from build123d import *

# Parameters (mm, degrees)
SKETCH_1_W         = 10
SKETCH_1_H         = 10
EXTRUDE_1_DEPTH    = 1
EXTRUDE_2_DEPTH    = 1
SKETCH_4_W         = 12
SKETCH_4_H         = 17
EXTRUDE_4_DEPTH    = 1
SKETCH_5_W         = 12
SKETCH_5_H         = 17
EXTRUDE_5_DEPTH    = 1
HOLE_WIZARD_M2_1_D = 1.6


with BuildPart() as part:
    # 草图1 → 凸台-拉伸1 (new body)
    with BuildSketch(Plane(origin=(0, 0, 0), x_dir=(1, 0, 0), z_dir=(0, 1, 0))):
        with Locations((5, 5)):
            Rectangle(SKETCH_1_W, SKETCH_1_H)
    extrude(amount=EXTRUDE_1_DEPTH)

    # 草图2 → 凸台-拉伸2 (add)
    with BuildSketch(Plane.ZY):
        with BuildLine():
            Line((-9.5, 6.5), (-10, 6.5))
            Line((-10, 6.5), (-10, 0))
            Line((-10, 0), (0, 0))
            Line((0, 0), (0, 6.5))
            Line((0, 6.5), (-0.5, 6.5))
            ThreePointArc((-0.5, 6.5), (-5, 2), (-9.5, 6.5))
        make_face()
    extrude(amount=EXTRUDE_2_DEPTH)

    # 草图4 → 凸台-拉伸4 (add)
    with BuildSketch(Plane.XY):
        with Locations((5, 8.5)):
            Rectangle(SKETCH_4_W, SKETCH_4_H)
    extrude(amount=EXTRUDE_4_DEPTH)

    # 草图5 → 凸台-拉伸5 (add)
    with BuildSketch(Plane(origin=(0, 0, -10), x_dir=(-1, 0, 0), z_dir=(0, 0, -1))):
        with Locations((-5, 8.5)):
            Rectangle(SKETCH_5_W, SKETCH_5_H)
    extrude(amount=EXTRUDE_5_DEPTH)

    # M2 螺纹孔1 (through all)
    with Locations(Plane(origin=(0, 0, -11), x_dir=(-1, 0, 0), z_dir=(0, 0, -1))):
        with Locations((-9, 15.5), (-1, 15.5)):
            Hole(HOLE_WIZARD_M2_1_D / 2)


solid = part.part
Geometry: final body of the model. Coordinates: model frame, mm. A direction names the side the tool comes from. Give positions to 0.01 mm unless a question says otherwise; leave off trailing zeros. Order: outer loops, then holes, each group sorted by start corner. A loop starts at its lowest first (then second) coordinate and runs counter-clockwise, first axis right, second up. Notation, with made-up numbers: (-30, 26.5) - (18, 26.5) arc R27 cw to (18, 62.5) - close; hole circle Ø6 at (40.25, 48.5). An arc over 180 degrees is marked (long way). Use CSV: the item, a comma, the result in double quotes.
1. Section query A-A (x = 1). Output: boundary loops of the cut face in (y, z), plus the area to 3 significant figures.
Answers below:
outline,"(0, -11) - (14.7, -11) - (14.7, -10) - (1, -10) - (1, 0) - (14.7, 0) - (14.7, 1) - (0, 1) - close; (16.3, -11) - (17, -11) - (17, -10) - (16.3, -10) - close; (16.3, 0) - (17, 0) - (17, 1) - (16.3, 1) - close"
area,"40.8 mm2"
2. Contact query for a flat-ended pin moving along its axis: pin 1 (0.5 mm diameter, centred on y = 0.5, z = -3, fed in from +X). Output: stop coordinate, or through.
Answers below:
pin 1,"x = 10"
3. Section query D-D (z = -0.25). Output: boundary loops of the cut face in (x, y).
Answers below:
outline,"(-1, 0) - (10, 0) - (10, 1) - (0, 1) - (0, 6.5) - (-1, 6.5) - close"
4. Access query for faces 1 (the face through (0, 2, -6.2)), 2 (the face through (5.1, 17, -10.5)), 3 (the face through (10, 0.5, -4.9)). Directions: +Z, -Z, +X, -X, +Y, -Y. A direction counts if a zero-diameter tool reaches every point of the face in a straight line with its end or side. Return the directions, or none.
Answers below:
face 1,"+X, +Y"
face 2,"+Z, -Z, +X, -X, +Y"
face 3,"+X, +Y, -Y"
5. Section query C-C (x = 10.25). Output: boundary loops of the cut face in (y, z).
Answers below:
outline,"(0, -11) - (17, -11) - (17, -10) - (0, -10) - close; (0, 0) - (17, 0) - (17, 1) - (0, 1) - close"
6. Material intervals for line 1 along Z through (x, y) = (0, 10.25); line 2 along Y through (x, z) = (1, -10.7); line 3 along Y through (x, z) = (0.25, -0.25), sorted ascending. Write a range as from..to.
Answers below:
line 1,"-11..-10, 0..1"
line 2,"0..14.7, 16.3..17"
line 3,"0..1"
7. Section query B-B (y = 15.5). Output: boundary loops of the cut face in (x, z), plus the area to 3 significant figures.
Answers below:
outline,"(-1, -11) - (0.2, -11) - (0.2, -10) - (-1, -10) - close; (-1, 0) - (0.2, 0) - (0.2, 1) - (-1, 1) - close; (1.8, -11) - (8.2, -11) - (8.2, -10) - (1.8, -10) - close; (1.8, 0) - (8.2, 0) - (8.2, 1) - (1.8, 1) - close; (9.8, -11) - (11, -11) - (11, -10) - (9.8, -10) - close; (9.8, 0) - (11, 0) - (11, 1) - (9.8, 1) - close"
area,"17.6 mm2"
8. Mould query, pull axis Y, two halves, no side actions, for faces 4 (the face through (5, 0, -5)), 5 (the face through (-0.5, 2, -4.9)), 6 (the face through (-1, 2.7, -2.2)), 7 (the face through (8.37, 15.01, -10.49)). Classes: +Y half, -Y half, draft (parallel to the pull), parting line (faces both ways), or undercut.
Answers below:
face 4,"-Y half"
face 5,"+Y half"
face 6,"draft"
face 7,"undercut"
